Geometry: final body of the model. Coordinates: model frame, mm. A direction names the side the tool comes from. Round coordinates to 2 decimals unless told otherwise and drop trailing zeros. Loops run counter-clockwise (first coordinate to the right, second up) from the corner with the lowest first, then second, coordinate; pieces in that order, holes last. Notation, with made-up numbers: (16.25, 3) - (34.25, 3) arc R25 cw to (34.25, 15) - close; hole circle Ø1 at (-28, 40). An arc over 180 degrees is marked (long way). Write item = value, one per line. Start each with the question number.
Item 1: Section B-B (z = -6.1). Return loops of the section in (x, y).
Item 2: First-contact query: pin 1 (6.5 mm diameter, centred on x = 16, z = -24, fed in from +Y); pin 2 (4 mm diameter, centred on x = 9, z = -17.5, fed in from +Y). Flat tips, straight axial feed; report the tip coordinate or a pass-through.
Item 3: Access query for faces 1 (the cylindrical face through (5.525, 23.664, -35.714)), 2 (the cylindrical face through (25.613, 48.986, -31.761)). Directions: +Z, -Z, +X, -X, +Y, -Y. A direction counts if a zero-diameter tool reaches every point of the face in a straight line with its end or side. Return the directions, or none.
Item 4: Draft query along Z for faces 3 (the cylindrical face through (35.77, 23.66, -5.41)), 4 (the flat face through (16, 48, -32)), 5 (the cylindrical face through (23.51, 60.85, -20.26)), 6 (the flat face through (21, 24, 0)). Return one class per face: pulls with the +Z half, pulls with the -Z half, needs draft (parallel to the pull), parting line crosses it, or undercut.
Item 5: Section C-C (x = 37.1). Return loops of the section in (y, z), plus the area to 3 significant figures.
Item 6: Line query: line 1 (Z direction, x = 6, y = 27); line 2 (X direction, y = 12, z = -6); line 3 (X direction, y = 40, z = -6.5). Output: solid intervals per line, ascending. Write a range as from..to.
Item 7: Section D-D (x = 21.4). Return loops of the section in (y, z), plus the area to 3 significant figures.
Item 8: Section A-A (y = 37). Return loops of the section in (x, z), plus the area to 3 significant figures.
from build123d import *

# Parameters (mm, degrees)
SKETCH1_W           = 43.2
SKETCH1_H           = 43.2
SKETCH1_R           = 1.5
BOSS_EXTRUDE1_DEPTH = 48
CHAMFER1_SIZE       = 2
SKETCH2_R           = 11
BOSS_EXTRUDE2_DEPTH = 2
SKETCH3_R           = 2.5
BOSS_EXTRUDE3_DEPTH = 24


with BuildPart() as part:
    # Sketch1 → Boss-Extrude1 (new body)
    with BuildSketch(Plane(origin=(0, 0, 0), x_dir=(1, 0, 0), z_dir=(0, 1, 0))):
        with Locations((21.6, 21.6)):
            Rectangle(SKETCH1_W, SKETCH1_H)
        with Locations(Location((6.1, 37.1, 0), (0, 0, 270))):
            Circle(SKETCH1_R, mode=Mode.SUBTRACT)
        with Locations(Location((37.1, 37.1, 0), (0, 0, 270))):
            Circle(SKETCH1_R, mode=Mode.SUBTRACT)
        with Locations(Location((37.1, 6.1, 0), (0, 0, 270))):
            Circle(SKETCH1_R, mode=Mode.SUBTRACT)
        with Locations(Location((6.1, 6.1, 0), (0, 0, 270))):
            Circle(SKETCH1_R, mode=Mode.SUBTRACT)
    extrude(amount=BOSS_EXTRUDE1_DEPTH)

    # Chamfer1
    chamfer1_edges = [part.edges().sort_by_distance(p)[0] for p in [
        (0, 24, -43.2),
        (43.2, 24, -43.2),
        (43.2, 24, 0),
        (0, 24, 0),
    ]]
    chamfer(chamfer1_edges, length=CHAMFER1_SIZE)

    # Sketch2 → Boss-Extrude2 (add)
    with BuildSketch(Plane(origin=(0, 48, 0), x_dir=(1, 0, 0), z_dir=(0, 1, 0))):
        with Locations(Location((21.4, 21.6, 0), (0, 0, 90))):
            Circle(SKETCH2_R)
    extrude(amount=BOSS_EXTRUDE2_DEPTH)

    # Sketch3 → Boss-Extrude3 (add)
    with BuildSketch(Plane(origin=(0, 48, 0), x_dir=(1, 0, 0), z_dir=(0, 1, 0))):
        with Locations(Location((21.4, 21.6, 0), (0, 0, 270))):
            Circle(SKETCH3_R)
    extrude(amount=BOSS_EXTRUDE3_DEPTH)


solid = part.part
Taken from the geometry:
q1.outline = (0, 0) - (4.6, 0) - (4.6, 48) - (0, 48) - close; (7.6, 0) - (35.6, 0) - (35.6, 48) - (7.6, 48) - close; (38.6, 0) - (43.2, 0) - (43.2, 48) - (38.6, 48) - close
q2.pin_1 = 50
q2.pin_2 = 48
q3.face_1 = +Y, -Y
q3.face_2 = +Y
q4.face_3 = undercut
q4.face_4 = needs draft
q4.face_5 = parting line crosses it
q4.face_6 = pulls with the +Z half
q5.outline = (0, -43.2) - (48, -43.2) - (48, -38.6) - (0, -38.6) - close; (0, -35.6) - (48, -35.6) - (48, -7.6) - (0, -7.6) - close; (0, -4.6) - (48, -4.6) - (48, 0) - (0, 0) - close
q5.area = 1,790 mm^2
q6.line_1 = -43.2..-38.6, -35.6..-7.6, -4.6..0
q6.line_2 = 0..4.6, 7.6..35.6, 38.6..43.2
q6.line_3 = 0..4.65, 7.55..35.65, 38.55..43.2
q7.outline = (0, -43.2) - (48, -43.2) - (48, -32.6) - (50, -32.6) - (50, -24.1) - (72, -24.1) - (72, -19.1) - (50, -19.1) - (50, -10.6) - (48, -10.6) - (48, 0) - (0, 0) - close
q7.area = 2,230 mm^2
q8.outline = (0, -41.2) - (2, -43.2) - (41.2, -43.2) - (43.2, -41.2) - (43.2, -2) - (41.2, 0) - (2, 0) - (0, -2) - close; hole circle Ø3 at (6.1, -37.1); hole circle Ø3 at (6.1, -6.1); hole circle Ø3 at (37.1, -37.1); hole circle Ø3 at (37.1, -6.1)
q8.area = 1,830 mm^2
